from build123d import *

# Parameters (mm, degrees)
F0_R      = 47.751218
F1_DEPTH  = 152.4
F2_R      = 40.626072
F3_DEPTH  = 115.57
F4_W      = 88.883296
F4_H      = 24.363942
F5_DEPTH  = 63.5
F6_W      = 25.266318
F6_H      = 97.455788
F7_DEPTH  = 8.382
F8_W      = 25.266318
F8_H      = 11.73079
F9_DEPTH  = 25.4
F10_W     = 25.266318
F10_H     = 8.8453
F11_DEPTH = 25.4


with BuildPart() as f1:
    # F0 (on Top) → F1 (new body)
    with BuildSketch(Plane.XY):
        Circle(F0_R)
    extrude(amount=F1_DEPTH)

    # F2 (on face) → F3 (cut)
    with BuildSketch(Plane.XY.offset(152.4)):
        Circle(F2_R)
    extrude(amount=-F3_DEPTH, mode=Mode.SUBTRACT)

    # F4 (on Front) → F5 (join)
    with BuildSketch(Plane.XZ):
        with Locations((0, 64.04309)):
            Rectangle(F4_W, F4_H)
    extrude(amount=-F5_DEPTH)

    # F6 (on face) → F7 (join)
    with BuildSketch(Plane(origin=(0, 63.5, 0), x_dir=(-1, 0, 0), z_dir=(0, 1, 0))):
        with Locations((-0.676776, 100.589013)):
            Rectangle(F6_W, F6_H)
    extrude(amount=F7_DEPTH)

    # F8 (on face) → F9 (join)
    with BuildSketch(Plane(origin=(0, 71.882, 0), x_dir=(-1, 0, 0), z_dir=(0, 1, 0))):
        with Locations((-0.676776, 143.451512)):
            Rectangle(F8_W, F8_H)
    extrude(amount=F9_DEPTH)

    # F10 (on face) → F11 (join)
    with BuildSketch(Plane(origin=(0, 0, 137.586117), x_dir=(1, 0, 0), z_dir=(0, 0, -1))):
        with Locations((0.676776, -92.85935)):
            Rectangle(F10_W, F10_H)
    extrude(amount=F11_DEPTH)


solid = f1.part
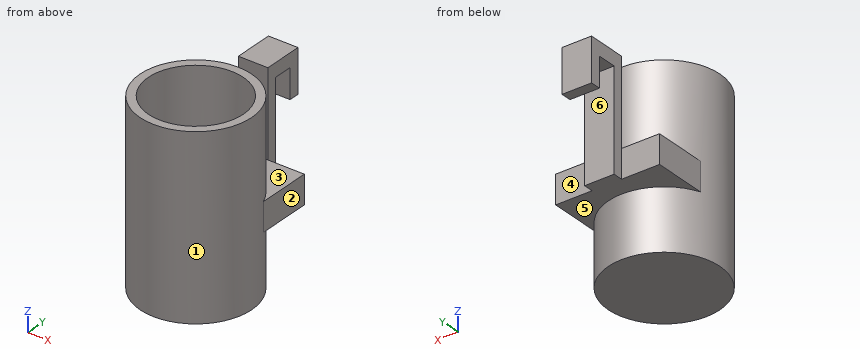
For this review, take the finished solid that the model builds, in its own axes (mm). Face numbers are marked on the shaded views. A direction names the side the tool comes from. Give positions to 0.01 mm unless a question says otherwise; leave off trailing zeros. Order: outer loops, then holes, each group sorted by start corner. A loop starts at its lowest first (then second) coordinate and runs counter-clockwise, first axis right, second up. Notation, with made-up numbers: (23, 40.25) -> (69, 40.25) arc R25 cw to (69, 64.25) -> close; hole circle Ø7 at (18.5, 41). An arc over 180 degrees is marked (long way). Write item = value, one per line.
1) For the marked faces 1, 2 and 3, list the 3-axis set-ups (+Z, -Z, +X, -X, +Y, -Y) from which the entire face can be reached by the end or side of a thin tool; tool diameter is ignored.
Findings:
face_1 = none
face_2 = +Z, -Z, +X, +Y
face_3 = +Z
2) Draft analysis for pull direction Y (two halves, no side actions). For the marked faces 4, 5 and 6, state which applies: pulls with the +Y half, pulls with the -Y half, needs draft (parallel to the pull), parting line crosses it, or undercut.
Findings:
face_4 = pulls with the +Y half
face_5 = needs draft
face_6 = undercut
3) To check wall thickness, follow L1, parallel to Y at x = 0, z = 114; L2, parallel to Z at x = -12, y = 10; L3, parallel to Y at x = 5.5, z = 139. State the ranges of each line that lie inside material, in increasing order. Write a range as from..to.
Findings:
L1 = -47.75..-40.63, 40.63..47.75, 63.5..71.88, 88.44..97.28
L2 = 0..36.83, 51.86..76.23
L3 = -47.43..-40.25, 40.25..47.43, 63.5..97.28
4) Insertion check: pin 1 (2 mm diameter, centred on x = -12, z = 94.5, fed in from +Y); pin 2 (1 mm diameter, centred on y = 2, z = 108.5, fed in from +X); pin 3 (12 mm diameter, centred on y = 36, z = 58.5, fed in from +X). Each pin has a flat end and moves straight along its axis. Give the tip position at first contact, or say it passes through.
Findings:
pin_1 = 71.88
pin_2 = 47.73
pin_3 = 44.44
5) We need section A-A, the plane z = 69.5. Give the boundary of the cut face in (x, y), and give its area (3 significant figures).
Findings:
outline = (-44.44, 17.47) arc R47.75 ccw (long way) to (44.44, 17.47) -> (44.44, 63.5) -> (13.31, 63.5) -> (13.31, 71.88) -> (-11.96, 71.88) -> (-11.96, 63.5) -> (-44.44, 63.5) -> close; hole (-40.63, 0) arc R40.63 ccw to (40.63, 0) -> close
area = 6,920 mm^2
6) We need section B-B, the plane x = 0. Give the boundary of the cut face in (y, z).
Findings:
outline = (-47.75, 0) -> (47.75, 0) -> (47.75, 51.86) -> (71.88, 51.86) -> (71.88, 137.59) -> (88.44, 137.59) -> (88.44, 112.19) -> (97.28, 112.19) -> (97.28, 149.32) -> (63.5, 149.32) -> (63.5, 76.23) -> (47.75, 76.23) -> (47.75, 152.4) -> (40.63, 152.4) -> (40.63, 76.23) -> (0, 76.23) -> (0, 51.86) -> (40.63, 51.86) -> (40.63, 36.83) -> (-40.63, 36.83) -> (-40.63, 152.4) -> (-47.75, 152.4) -> close
7) We need section C-C, the plane z = 100.5. Give the boundary of the cut face in (x, y), and give its area (3 significant figures).
Findings:
outline = circle Ø95.5 at (0, 0); (-11.96, 63.5) -> (13.31, 63.5) -> (13.31, 71.88) -> (-11.96, 71.88) -> close; hole circle Ø81.25 at (0, 0)
area = 2,190 mm^2
8) We need section D-D, the plane y = -18. Give the boundary of the cut face in (x, z), and give its area (3 significant figures).
Findings:
outline = (-44.23, 0) -> (44.23, 0) -> (44.23, 152.4) -> (36.42, 152.4) -> (36.42, 36.83) -> (-36.42, 36.83) -> (-36.42, 152.4) -> (-44.23, 152.4) -> close
area = 5,060 mm^2
